Read the model definition and answer for the solid it produces. Units are mm, in the model's axes. A direction names the side the tool comes from. Round coordinates to 2 decimals unless told otherwise and drop trailing zeros. Loops run counter-clockwise (first coordinate to the right, second up) from the corner with the lowest first, then second, coordinate; pieces in that order, holes last. Notation, with made-up numbers: M 57.25,87.25 L 101.25,87.25 A21 cw 101.25,94.25 Z; hole C 21,27.5 d5. An arc over 180 degrees is marked long. Answer as CSV lines item,"result".
```python
from build123d import *

# Parameters (mm, degrees)
BASE_FLANGE1_DEPTH                            = 3.175
SKETCHED_START                                = -39.6875
SKETCHED_BEND2_DEPTH                          = 79.375
SKETCHED_BEND2_2_DEPTH                        = 79.375
SKETCHED_START_2                              = 554.168566106
SKETCHED_BEND2_3_DEPTH                        = 4.831433894
EXTRUDE3_DEPTH                                = 1.5748
F_9_0_196_DIAMETER_HOLE1_D                    = 4.9784
F_9_0_196_DIAMETER_HOLE1_CSINK_D              = 5.715
F_9_0_196_DIAMETER_HOLE1_CSINK_ANGLE          = 90
CHAMFER1_SIZE                                 = 0.889
F_0_116_DIAMETER_HOLE1_D                      = 2.9464
CSK_FOR_4_FLAT_HEAD_MACHINE_SCREW1_AT_2_COUNT = 2
CSK_FOR_4_FLAT_HEAD_MACHINE_SCREW1_AT_2_PITCH = 16.160968319
CSK_FOR_4_FLAT_HEAD_MACHINE_SCREW1_AT_3_COUNT = 2
CSK_FOR_4_FLAT_HEAD_MACHINE_SCREW1_AT_3_PITCH = 11.43
CSK_FOR_4_FLAT_HEAD_MACHINE_SCREW1_AT_4_COUNT = 2
CSK_FOR_4_FLAT_HEAD_MACHINE_SCREW1_AT_4_PITCH = 18.194716953


with BuildPart() as part:
    # Base-Flange1: sheet metal written as solids
    # Sketch1 → Base-Flange1 (new body)
    with BuildSketch(Plane.XY):
        with BuildLine():
            Line((93.6498, 4.974967896), (552.323, 44.950411579))
            Line((552.323, 44.950411579), (552.323, 43.6499))
            ThreePointArc((552.323, 43.6499), (553.48356009, 40.84806009), (556.2854, 39.6875))
            Line((556.2854, 39.6875), (568.198, 39.6875))
            ThreePointArc((568.198, 39.6875), (572.688128061, 37.827628061), (574.548, 33.3375))
            Line((574.548, 33.3375), (574.548, -33.3375))
            ThreePointArc((574.548, -33.3375), (572.688128061, -37.827628061), (568.198, -39.6875))
            Line((568.198, -39.6875), (556.2854, -39.6875))
            ThreePointArc((556.2854, -39.6875), (553.48356009, -40.84806009), (552.323, -43.6499))
            Line((552.323, -43.6499), (552.323, -46.531181284))
            Line((552.323, -46.531181284), (93.6498, -6.555737601))
            Line((93.6498, -6.555737601), (93.6498, 4.974967896))
        make_face()
    extrude(amount=-BASE_FLANGE1_DEPTH)

    # Sketched Bend2: read off the stored shape, not the designer's step
    # Sketched Bend2 outline → Sketched Bend2 (cut)
    with BuildSketch(Plane(origin=(0, 0, 0), x_dir=(1, 0, 0), z_dir=(0, 1, 0)).offset(SKETCHED_START)):
        with BuildLine():
            ThreePointArc((556.949152286, 3.175), (559.367160247, 2.270079642), (560.596949567, 0))
            Line((560.596949567, 0), (574.548, 0))
            Line((574.548, 0), (574.548, 3.175))
            Line((574.548, 3.175), (556.949152286, 3.175))
        make_face()
    extrude(amount=SKETCHED_BEND2_DEPTH, mode=Mode.SUBTRACT)

    # Sketched Bend2 2 outline → Sketched Bend2 2 (add)
    with BuildSketch(Plane(origin=(0, 0, 0), x_dir=(1, 0, 0), z_dir=(0, 1, 0)).offset(SKETCHED_START)):
        with BuildLine():
            Line((557.455219193, -0.463724883), (558.718115569, -14.89869652))
            Line((558.718115569, -14.89869652), (561.881033736, -14.621977036))
            Line((561.881033736, -14.621977036), (560.618137359, -0.187005399))
            ThreePointArc((560.618137359, -0.187005399), (560.608738158, -0.09336734), (560.596949567, 0))
            Line((560.596949567, 0), (556.949152286, 0))
            ThreePointArc((556.949152286, 0), (557.292352112, -0.133463113), (557.455219193, -0.463724883))
        make_face()
    extrude(amount=SKETCHED_BEND2_2_DEPTH)

    # Sketched Bend2 3 outline → Sketched Bend2 3 (cut)
    with BuildSketch(Plane(origin=(0, 0, 0), x_dir=(0, 1, 0), z_dir=(0.9961946980917459, 0, -0.0871557427476548)).offset(SKETCHED_START_2)):
        with BuildLine():
            Line((39.6875, 63.537494831), (33.3375, 63.53749483))
            ThreePointArc((33.3375, 63.53749483), (37.827628061, 61.677622891), (39.6875, 57.18749483))
            Line((39.6875, 57.18749483), (39.6875, 63.537494831))
        make_face()
        with BuildLine():
            ThreePointArc((-39.6875, 57.18749483), (-37.827628061, 61.677622891), (-33.3375, 63.53749483))
            Line((-33.3375, 63.53749483), (-39.6875, 63.537494831))
            Line((-39.6875, 63.537494831), (-39.6875, 57.18749483))
        make_face()
    extrude(amount=SKETCHED_BEND2_3_DEPTH, mode=Mode.SUBTRACT)

    # Sketch6 → Extrude3 (add)
    with BuildSketch(Plane.XY):
        Polygon((93.6498, 2.425339339), (93.6498, 8.162003592), (552.323, 48.137447275), (552.323, 42.400783022), align=None)
    extrude(amount=-EXTRUDE3_DEPTH)

    # #9 (0.196) Diameter Hole1 (through all)
    with Locations(Plane(origin=(553.180458015, 0, -48.39701896), x_dir=(0.08715574274765482, 0, 0.9961946980917459), z_dir=(-0.9961946980917459, 0, 0.08715574274765482))):
        with Locations((56.40009483, 9.525), (56.40009483, 28.575), (56.40009483, -28.575), (56.40009483, -9.525)):
            CounterSinkHole(F_9_0_196_DIAMETER_HOLE1_D / 2, F_9_0_196_DIAMETER_HOLE1_CSINK_D / 2, counter_sink_angle=F_9_0_196_DIAMETER_HOLE1_CSINK_ANGLE)

    # Chamfer1
    chamfer1_edges = [part.edges().sort_by_distance(p)[0] for p in [
        (322.9864, -26.543459443, -3.175),
    ]]
    chamfer(chamfer1_edges, length=CHAMFER1_SIZE)

    # 0.116_ Diameter Hole1 (through all)
    with Locations(Plane(origin=(0, 0, -3.175), x_dir=(-1, 0, 0), z_dir=(0, 0, -1))):
        with Locations((-381, 23.8125), (-381, -23.8125), (-203.2, 9.525), (-203.2, -9.525), (-97.6376, 0), (-545.973, 36.5125), (-545.973, -36.5125)):
            Hole(F_0_116_DIAMETER_HOLE1_D / 2)

    # Sketch15 → CSK for #4 Flat Head Machine Screw1 (revolve, cut)
    with BuildSketch(Plane(origin=(170.0784, 7.112, 0), x_dir=(0, -1, 0), z_dir=(1, 0, 0))):
        Polygon((0, 0), (0, 3.175), (1.4732, 3.175), (1.4732, 1.592454986), (2.8575, 0), align=None)
    csk_for_4_flat_head_machine_screw1 = revolve(axis=Axis((170.0784, 7.112, 6.35), (0, 0, -1)), mode=Mode.SUBTRACT)

    # CSK for #4 Flat Head Machine Screw1 at 2: CSK for #4 Flat Head Machine Screw1 ×2
    with Locations(*[Vector(0.06286752006193388, -0.998021880983209, 0) * (i * CSK_FOR_4_FLAT_HEAD_MACHINE_SCREW1_AT_2_PITCH) for i in range(1, CSK_FOR_4_FLAT_HEAD_MACHINE_SCREW1_AT_2_COUNT)]):
        add(csk_for_4_flat_head_machine_screw1, mode=Mode.SUBTRACT)

    # CSK for #4 Flat Head Machine Screw1 at 3: CSK for #4 Flat Head Machine Screw1 ×2
    with Locations(*[(i * CSK_FOR_4_FLAT_HEAD_MACHINE_SCREW1_AT_3_PITCH, 0, 0) for i in range(1, CSK_FOR_4_FLAT_HEAD_MACHINE_SCREW1_AT_3_COUNT)]):
        add(csk_for_4_flat_head_machine_screw1, mode=Mode.SUBTRACT)

    # CSK for #4 Flat Head Machine Screw1 at 4: CSK for #4 Flat Head Machine Screw1 ×2
    with Locations(*[Vector(0.4048427914006695, -0.9143863047153069, 0) * (i * CSK_FOR_4_FLAT_HEAD_MACHINE_SCREW1_AT_4_PITCH) for i in range(1, CSK_FOR_4_FLAT_HEAD_MACHINE_SCREW1_AT_4_COUNT)]):
        add(csk_for_4_flat_head_machine_screw1, mode=Mode.SUBTRACT)


solid = part.part
```
1) Find section A-A, the plane x = 300. Give the vertices of the cut face in (y, z) (3 decimals), then the cut area to 3 significant figures.
Evaluation:
outline,"M -24.54,-2.286 L -23.648,-3.175 L 22.959,-3.175 L 22.959,-1.575 L 26.146,-1.575 L 26.146,0 L -24.54,0 Z"
area,"155 mm^2"
2) Each of these flat-tipped pins is pushed along its axis until it touches: P1, Ø8, axis at x = 191, z = 1.5, coming from the -Y side; P2, Ø3.5, axis at x = 171.09, y = -9.02, coming from the -Z side (3 decimals); P3, Ø10, axis at x = 272.5, y = -18, coming from the +Z side; P4, Ø3.5, axis at y = 46.5, z = -1.5, coming from the +X side. Where does it stop, or does it pass through?
Evaluation:
P1,"stops at y = -15.36"
P2,"stops at z = -3.175"
P3,"stops at z = 0"
P4,"stops at x = 552.32"
3) Find section C-C, the plane x = 219. Give the vertices of the cut face in (y, z) (3 decimals).
Evaluation:
outline,"M -17.481,-2.286 L -16.588,-3.175 L 15.9,-3.175 L 15.9,-1.575 L 19.087,-1.575 L 19.087,0 L -17.481,0 Z"
4) Determine the mould class of faces 1 (the flat face through (326.197, -26.383, -2.724)), 2 (the flat face through (380, 1, 0)), 3 (the flat face through (319.78, 27.87, -0.78)) for opening direction Y: released by +Y, released by -Y, zero draft, split by the parting line, or undercut.
Evaluation:
face 1,"released by -Y"
face 2,"zero draft"
face 3,"released by +Y"
5) Find section B-B, the plane y = -18.5. Give the vertices of the cut face in (x, z) (3 decimals), then the cut area to 3 significant figures.
Evaluation:
outline,"M 230.697,-2.286 L 240.936,-3.175 L 556.949,-3.175 A3.683 ccw 560.597,0 A3.683 ccw 560.618,0.187 L 561.881,14.622 L 558.718,14.899 L 557.455,0.464 A0.508 cw 556.949,0 L 230.697,0 Z"
area,"1,090 mm^2"
6) A tool of negligible diameter and unlimited length cuts with its end or side. For faces 4 (the flat face through (326.197, -26.823, -1.127)), 5 (the flat face through (319.776, 24.683, -2.364)), from which of +Z, -Z, +X, -X, +Y, -Y can it reach the whole face along a straight path? Write none if from no direction.
Evaluation:
face 4,"+Z, -Z, -X, -Y"
face 5,"-Z, -X, +Y"
7) Straight lines are drawn through the part: line 1 (Y direction, x = 381, z = -1.8); line 2 (Z direction, x = 292.5, y = -21) (3 decimals); line 3 (X direction, y = 22.5, z = 0.25). For each, find the intervals that lie inside material, in ascending order.
Evaluation:
line 1,"y = -31.6 to -25.29, -22.34 to 22.34, 25.29 to 30.02"
line 2,"z = -3.175 to 0"
line 3,"x = 557.39 to 560.62"
